Part model, mm, in its own coordinate system. Round coordinates to 2 decimals unless told otherwise and drop trailing zeros. Loops run counter-clockwise (first coordinate to the right, second up) from the corner with the lowest first, then second, coordinate; pieces in that order, holes last.
1) Drop a flat-ended pin along its axis: P1, Ø10, axis at x = -27.15, y = -38.38, coming from the -Z side. Give the stop position or say it passes through.
2) Band-saw the part on A-A, the plane z = 2. Write the cut outline in (x, y).
3) Probe line 1 (Y direction, x = -9, z = 1.5); line 2 (Y direction, x = -7.5, z = 5.25); line 3 (Y direction, x = -63, z = 1.5). List the from-to ranges inside material, lowest first.
from build123d import *

# Parameters (mm, degrees)
F0_W           = 127
F0_H           = 444.5
F1_DEPTH       = 6.35
F4_D           = 7.7597
F4_DEPTH       = 9.525
F4_CSINK_D     = 17.78
F4_CSINK_ANGLE = 77
F4_TIP         = 2.3312490727
F5_R           = 3.17499


# Not quite as in the source:
# - a fillet or chamfer is up to 0.001 mm smaller than in the source, because OpenCascade refuses the exact size


with BuildPart() as f1:
    # F0 (on Top) → F1 (new body)
    with BuildSketch(Plane.XY):
        with Locations((-9.3688531779, 39.7230851987)):
            Rectangle(F0_W, F0_H)
    extrude(amount=F1_DEPTH)

    # F4
    with Locations(Plane(origin=(0, 0, 0), x_dir=(1, 0, 0), z_dir=(0, 0, -1))):
        with Locations((41.4311468221, -249.2730851987), (-9.3688531779, -230.2230851987), (-60.1688531779, -249.2730851987), (-9.3688531779, -194.2820851987), (-9.3688531779, -143.4820851987), (8.4111468221, 38.3819148013), (-27.1488531779, 38.3819148013)):
            CounterSinkHole(F4_D / 2, F4_CSINK_D / 2, depth=F4_DEPTH, counter_sink_angle=F4_CSINK_ANGLE)
            with Locations((0, 0, -(F4_DEPTH + F4_TIP / 2))):  # 118° drill point
                Cone(0, F4_D / 2, F4_TIP, mode=Mode.SUBTRACT)

    # F5 (radius 3.175 in the source; OpenCascade refuses exactly that, so slightly less here)
    f5_edges = [f1.edges().sort_by_distance(p)[0] for p in [
        (-9.368853, -182.526915, 6.35),
        (-9.368853, -182.526915, 0),
    ]]
    fillet(f5_edges, radius=F5_R)


solid = f1.part
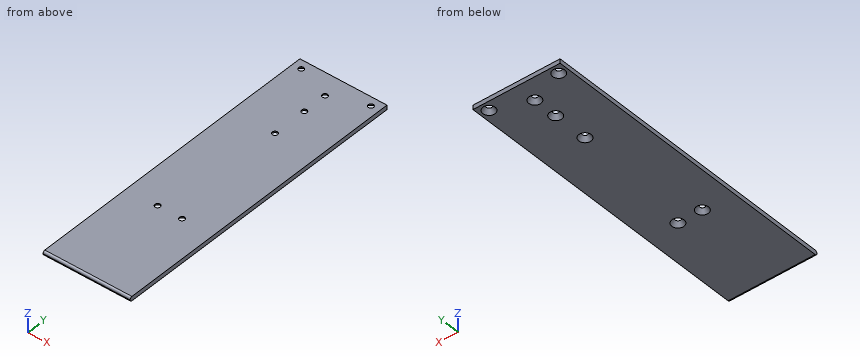
Reported:
1. P1: stops at z = 4.89
2. outline: (-72.87, -182.3) - (54.13, -182.3) - (54.13, 261.97) - (-72.87, 261.97) - close; hole circle Ø14.6 at (-60.17, 249.27); hole circle Ø14.6 at (-27.15, -38.38); hole circle Ø14.6 at (-9.37, 143.48); hole circle Ø14.6 at (-9.37, 194.28); hole circle Ø14.6 at (-9.37, 230.22); hole circle Ø14.6 at (8.41, -38.38); hole circle Ø14.6 at (41.43, 249.27)
3. line 1: y = -182.05 to 135.79, 151.17 to 186.59, 201.97 to 222.54, 237.91 to 261.97
3. line 2: y = -181.76 to 139.15, 147.81 to 189.95, 198.61 to 225.9, 234.55 to 261.97
3. line 3: y = -182.05 to 242.12, 256.43 to 261.97
